Input: part model. Units: mm. Frame: model coordinates. Face numbers are marked on the shaded views. Give positions to 0.01 mm unless a question says otherwise; leave off trailing zeros. Order: outer loops, then holes, each group sorted by start corner. A loop starts at its lowest first (then second) coordinate and runs counter-clockwise, first axis right, second up. Notation, with made-up numbers: (12.5, 22) - (22.5, 22) arc R23 ccw to (22.5, 38) - close; hole circle Ø9 at (13.25, 10.5). An arc over 180 degrees is marked (long way). Use a Markdown table: item, result.
Autodesk Fusion 360 part; units mm, degrees
sketch "スケッチ1" plane through (0, 0, 0) normal (0, 0, 1) x (1, 0, 0)
  circle A0 centre (0, 0) radius 2.45
  circle A1 centre (0, 0) radius 3.5
  line L0 (-3.5, 0) -> (3.5, 0) construction
  line L1 (0, 3.5) -> (0, -3.5) construction
  line L2 (-0.35, 2.4249) -> (0, 2.25)
  line L3 (0.35, 2.4249) -> (0, 2.25)
  line L4 (-0.35, 2.4249) -> (0.35, 2.4249) construction
  line L5 (0, 2.45) -> (0, 2.25) construction
  circle A2 centre (0, 0) radius 1.25
  line L6 (0, 3.5) -> (0, 18.5) construction
  line L7 (-2.75, 2.1651) -> (2.75, 2.1651) construction
  circle A3 centre (0, 16.6) radius 1.9
  line L8 (-1.9, 16.6) -> (1.9, 16.6) construction
  line L9 (-1.9, 16.6) -> (-2.75, 2.1651)
  line L10 (1.9, 16.6) -> (2.75, 2.1651)
  circle A4 centre (0, 17.3) radius 0.6
  circle A5 centre (0, 15.2) radius 0.6
  circle A6 centre (0, 13.1) radius 0.6
  circle A7 centre (0, 11) radius 0.6
  circle A8 centre (0, 8.9) radius 0.6
  circle A9 centre (0, 6.8) radius 0.6
  circle A10 centre (0, 0) radius 2.35
  dimension "d1" = 4.9
  dimension "d2" = 7
  dimension "d3" = 0.2
  dimension "d4" = 0.7
  dimension "d5" = 2.5
  dimension "d7" = 3.8
  dimension "d8" = 22
  dimension "d9" = 5.5
  dimension "d10" = 1.2
  dimension "d12" = 2.1
  dimension "d13" = 2.1
  dimension "d14" = 2.1
  dimension "d15" = 2.1
  dimension "d16" = 2.1
  dimension "d18" = 4.7
  dimension "d21" = 1.2
extrude "押し出し1" add sketch "スケッチ1" along normal blind 1 contours A0 L2 L3 A10 | A0 L2 L3 A10 | L2 L3 A10 | L2 L3 A10 | A1 | A1 A3 L9 L10 A5 | A3 A5 | A3 A5 picked at (0.9036, 16.1951) picked at (0, 14.6696)
extrude "押し出し2" add sketch "スケッチ1" along normal blind 1.5 contours A1 A3 L9 L10 A5 | A3 A5 | A3 A5 picked at (0.9036, 16.1951) picked at (0, 14.6696)
extrude "押し出し3" add sketch "スケッチ1" along normal blind 3 from surface at 1 contours A0 L2 L3 A10 | A0 L2 L3 A10 | L2 L3 A10 | L2 L3 A10 | A1
extrude "押し出し4" add sketch "スケッチ1" along normal blind 3 from surface at 4 contours A1
extrude "押し出し5" add sketch "スケッチ1" along normal blind 3 from surface at 4 contours A0 L2 L3 A10 | L2 L3 A10 picked at (-0.3559, 2.3522) picked at (0, 2.3161)
pattern_circular "C パターン1" count 22 over 360 about axis through (0, 0, 1.75) along (0, 0, 1) of "押し出し5"
extrude "押し出し6" cut sketch "スケッチ1" along normal blind 1.5 contours L2 L3 A10 | L2 L3 A10
chamfer "面取り1" distance 1 angle 45 1 edges at (-2.191, -0.8498, 1.5)
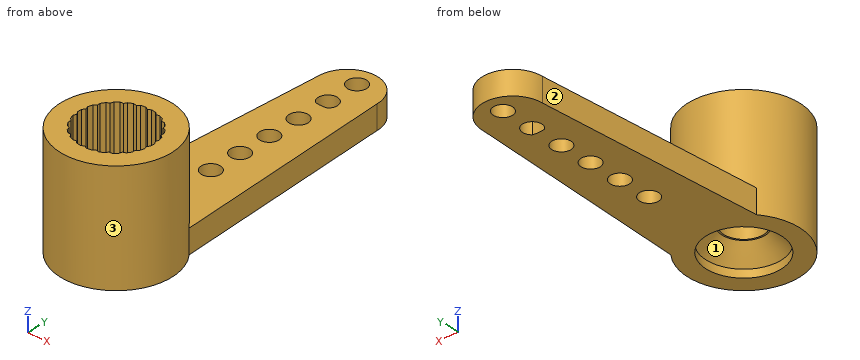
1. Pin query (flat end, axial travel): pin 1 (1.4 mm diameter, centred on x = 0.5, y = 0, fed in from -Z); pin 2 (4 mm diameter, centred on x = 0, y = 0, fed in from -Z); pin 3 (1.6 mm diameter, centred on x = 0, y = 13.1, fed in from +Z); pin 4 (4 mm diameter, centred on x = 0, y = 0, fed in from +Z). Return the tip coordinate at first contact, or that it passes through.
Response:
| item | result |
|---|---|
| pin 1 | passes through |
| pin 2 | stops at z = 0.85 |
| pin 3 | stops at z = 1.5 |
| pin 4 | stops at z = 4 |
2. Material intervals for line 1 along Z through (x, y) = (1, 13.25); line 2 along Y through (x, z) = (-0.75, 5); line 3 along Y through (x, z) = (2, 5.25), sorted ascending.
Response:
| item | result |
|---|---|
| line 1 | z = 0 to 1.5 |
| line 2 | y = -3.42 to -2.18, 2.18 to 3.42 |
| line 3 | y = -2.87 to -1.23, 1.23 to 2.87 |
3. Section query B-B (y = 13.5). Return loops of the section in (x, z), then the cut area to 3 significant figures.
Response:
| item | result |
|---|---|
| outline | (-2.08, 0) - (-0.45, 0) - (-0.45, 1.5) - (-2.08, 1.5) - close; (0.45, 0) - (2.08, 0) - (2.08, 1.5) - (0.45, 1.5) - close |
| area | 4.91 mm^2 |
4. Section query A-A (y = 6.8). Return loops of the section in (x, z), then the cut area to 3 significant figures.
Response:
| item | result |
|---|---|
| outline | (-2.48, 0) - (-0.6, 0) - (-0.6, 1.5) - (-2.48, 1.5) - close; (0.6, 0) - (2.48, 0) - (2.48, 1.5) - (0.6, 1.5) - close |
| area | 5.63 mm^2 |
5. Mould query, pull axis Y, two halves, no side actions, for the marked faces 1, 2 and 3. Classes: pulls with the +Y half, pulls with the -Y half, needs draft (parallel to the pull), parting line crosses it, or undercut.
Response:
| item | result |
|---|---|
| face 1 | undercut |
| face 2 | pulls with the +Y half |
| face 3 | parting line crosses it |
